from build123d import *

# Parameters (mm, degrees)
F0_R     = 1.5
F1_DEPTH = 3


with BuildPart() as f1:
    # F0 (on Top) → F1 (new body)
    with BuildSketch(Plane.XY):
        with BuildLine():
            ThreePointArc((26, 35), (22.464466, 26.464466), (31, 30))
            ThreePointArc((31, 30), (30.829629, 31.294095), (30.330127, 32.5))
            ThreePointArc((30.330127, 32.5), (28.5, 34.330127), (26, 35))
        make_face()
        with Locations((26, 30)):
            Circle(F0_R, mode=Mode.SUBTRACT)
        with BuildLine():
            ThreePointArc((30.330127, 32.5), (30.829629, 31.294095), (31, 30))
            ThreePointArc((31, 30), (22.464466, 26.464466), (26, 35))
            Line((26, 35), (-26, 35))
            ThreePointArc((-26, 35), (-22.464466, 33.535534), (-21, 30))
            ThreePointArc((-21, 30), (-27.294095, 25.170371), (-30.330127, 32.5))
            Line((-30.330127, 32.5), (-43.310889, 10.01666))
            ThreePointArc((-43.310889, 10.01666), (-37.686667, 12.34629), (-33.980762, 7.51666))
            ThreePointArc((-33.980762, 7.51666), (-37.686667, 2.687031), (-43.310889, 5.01666))
            Line((-43.310889, 5.01666), (-17.310889, -40.01666))
            ThreePointArc((-17.310889, -40.01666), (-14.274857, -32.687031), (-7.980762, -37.51666))
            ThreePointArc((-7.980762, -37.51666), (-9.445228, -41.052194), (-12.980762, -42.51666))
            Line((-12.980762, -42.51666), (12.980762, -42.51666))
            ThreePointArc((12.980762, -42.51666), (9.445228, -33.981127), (17.980762, -37.51666))
            ThreePointArc((17.980762, -37.51666), (17.810391, -38.810756), (17.310889, -40.01666))
            Line((17.310889, -40.01666), (43.310889, 5.01666))
            ThreePointArc((43.310889, 5.01666), (33.980762, 7.51666), (43.310889, 10.01666))
            Line((43.310889, 10.01666), (30.330127, 32.5))
        make_face()
        with Locations((-25.980762, -15)):
            Circle(F0_R, mode=Mode.SUBTRACT)
        with BuildLine():
            ThreePointArc((32.913325, 11.015246), (33.848011, 9.80077), (33.648709, 8.281274))
            Line((33.648709, 8.281274), (9.652561, -33.281274))
            ThreePointArc((9.652561, -33.281274), (8.43629, -34.213623), (6.91718, -34.011398))
            Line((6.91718, -34.011398), (5.99667, -33.477578))
            ThreePointArc((5.99667, -33.477578), (5.266988, -32.745787), (5, -31.747454))
            Line((5, -31.747454), (5, -30))
            ThreePointArc((5, -30), (0, -25), (-5, -30))
            Line((-5, -30), (-5, -31.747454))
            ThreePointArc((-5, -31.747454), (-5.266988, -32.745787), (-5.99667, -33.477578))
            Line((-5.99667, -33.477578), (-6.91718, -34.011398))
            ThreePointArc((-6.91718, -34.011398), (-8.43629, -34.213623), (-9.652561, -33.281274))
            Line((-9.652561, -33.281274), (-33.648709, 8.281274))
            ThreePointArc((-33.648709, 8.281274), (-33.848011, 9.80077), (-32.913325, 11.015246))
            Line((-32.913325, 11.015246), (-31.990768, 11.545521))
            ThreePointArc((-31.990768, 11.545521), (-30.992178, 11.811548), (-29.994102, 11.5436))
            Line((-29.994102, 11.5436), (-28.480762, 10.669873))
            ThreePointArc((-28.480762, 10.669873), (-21.650635, 12.5), (-23.480762, 19.330127))
            Line((-23.480762, 19.330127), (-24.994102, 20.203854))
            ThreePointArc((-24.994102, 20.203854), (-25.72519, 20.934239), (-25.994098, 21.932057))
            Line((-25.994098, 21.932057), (-25.996145, 22.996152))
            ThreePointArc((-25.996145, 22.996152), (-25.411722, 24.412853), (-23.996149, 25))
            Line((-23.996149, 25), (23.996149, 25))
            ThreePointArc((23.996149, 25), (25.411722, 24.412853), (25.996145, 22.996152))
            Line((25.996145, 22.996152), (25.994098, 21.932057))
            ThreePointArc((25.994098, 21.932057), (25.72519, 20.934239), (24.994102, 20.203854))
            Line((24.994102, 20.203854), (23.480762, 19.330127))
            ThreePointArc((23.480762, 19.330127), (21.650635, 12.5), (28.480762, 10.669873))
            Line((28.480762, 10.669873), (29.994102, 11.5436))
            ThreePointArc((29.994102, 11.5436), (30.992178, 11.811548), (31.990768, 11.545521))
            Line((31.990768, 11.545521), (32.913325, 11.015246))
        make_face(mode=Mode.SUBTRACT)
        with Locations((0, -30)):
            Circle(F0_R, mode=Mode.SUBTRACT)
        with Locations((25.980762, -15)):
            Circle(F0_R, mode=Mode.SUBTRACT)
        with Locations((-25.980762, 15)):
            Circle(F0_R, mode=Mode.SUBTRACT)
        with Locations((25.980762, 15)):
            Circle(F0_R, mode=Mode.SUBTRACT)
        with Locations((0, 30)):
            Circle(F0_R, mode=Mode.SUBTRACT)
        with BuildLine():
            ThreePointArc((43.980762, 7.51666), (43.810391, 8.810756), (43.310889, 10.01666))
            ThreePointArc((43.310889, 10.01666), (33.980762, 7.51666), (43.310889, 5.01666))
            ThreePointArc((43.310889, 5.01666), (43.810391, 6.222565), (43.980762, 7.51666))
        make_face()
        with Locations((38.980762, 7.51666)):
            Circle(F0_R, mode=Mode.SUBTRACT)
        with BuildLine():
            ThreePointArc((-21, 30), (-22.464466, 33.535534), (-26, 35))
            ThreePointArc((-26, 35), (-28.5, 34.330127), (-30.330127, 32.5))
            ThreePointArc((-30.330127, 32.5), (-27.294095, 25.170371), (-21, 30))
        make_face()
        with Locations((-26, 30)):
            Circle(F0_R, mode=Mode.SUBTRACT)
        with BuildLine():
            ThreePointArc((12.980762, -42.51666), (15.480762, -41.846788), (17.310889, -40.01666))
            ThreePointArc((17.310889, -40.01666), (17.810391, -38.810756), (17.980762, -37.51666))
            ThreePointArc((17.980762, -37.51666), (9.445228, -33.981127), (12.980762, -42.51666))
        make_face()
        with Locations((12.980762, -37.51666)):
            Circle(F0_R, mode=Mode.SUBTRACT)
        with BuildLine():
            ThreePointArc((-33.980762, 7.51666), (-37.686667, 12.34629), (-43.310889, 10.01666))
            ThreePointArc((-43.310889, 10.01666), (-43.980762, 7.51666), (-43.310889, 5.01666))
            ThreePointArc((-43.310889, 5.01666), (-37.686667, 2.687031), (-33.980762, 7.51666))
        make_face()
        with Locations((-38.980762, 7.51666)):
            Circle(F0_R, mode=Mode.SUBTRACT)
        with BuildLine():
            ThreePointArc((-17.310889, -40.01666), (-15.480762, -41.846788), (-12.980762, -42.51666))
            ThreePointArc((-12.980762, -42.51666), (-9.445228, -41.052194), (-7.980762, -37.51666))
            ThreePointArc((-7.980762, -37.51666), (-14.274857, -32.687031), (-17.310889, -40.01666))
        make_face()
        with Locations((-12.980762, -37.51666)):
            Circle(F0_R, mode=Mode.SUBTRACT)
    extrude(amount=F1_DEPTH)


solid = f1.part
Here's how the part is built. I have some questions about the finished solid (model axes, mm). A direction names the side the tool comes from. Round coordinates to 2 decimals unless told otherwise and drop trailing zeros. Write each loop counter-clockwise with the first axis right and the second up, starting at its lowest first coordinate (ties: lowest second). Pieces come first, ordered by that corner, then holes. Notation, with made-up numbers: (72, 74.5) -> (93, 74.5) arc R19 cw to (93, 88.5) -> close; hole circle Ø3 at (18, 53.25). An arc over 180 degrees is marked (long way). One line per item, written item: value.
1) Suppose I cut it at D-D on x = -19. List the corners of the cut face in (y, z) for me.
Filled sheet:
outline: (-37.09, 0) -> (-17.09, 0) -> (-17.09, 3) -> (-37.09, 3) -> close; (25, 0) -> (35, 0) -> (35, 3) -> (25, 3) -> close
2) Suppose I cut it at B-B on y = 0.5. List the corners of the cut face in (x, z) for me.
Filled sheet:
outline: (-40.7, 0) -> (-29.16, 0) -> (-29.16, 3) -> (-40.7, 3) -> close; (29.16, 0) -> (40.7, 0) -> (40.7, 3) -> (29.16, 3) -> close
3) Suppose I cut it at C-C on y = 15. List the corners of the cut face in (x, z) for me, plus the area to 3 significant figures.
Filled sheet:
outline: (-40.43, 0) -> (-27.48, 0) -> (-27.48, 3) -> (-40.43, 3) -> close; (-24.48, 0) -> (-20.98, 0) -> (-20.98, 3) -> (-24.48, 3) -> close; (20.98, 0) -> (24.48, 0) -> (24.48, 3) -> (20.98, 3) -> close; (27.48, 0) -> (40.43, 0) -> (40.43, 3) -> (27.48, 3) -> close
area: 98.7 mm2
4) For faces 1 (the face through (0, 25, 1)), 2 (the face through (36.91, 21.1, 1.48)), which set-ups out of +Z, -Z, +X, -X, +Y, -Y let a thin tool reach every point of the face, with its end or its side?
Filled sheet:
face 1: +Z, -Z
face 2: +Z, -Z, +X, +Y
5) If I drill on line 1 (X direction, y = 7, z = 2.2); line 2 (Y direction, x = -24, z = 1.45); line 3 (Y direction, x = 25, z = 1.8), over which ranges is the centre line in solid material (lowest first)? Write a range as [from, to].
Filled sheet:
line 1: x = [-43.95, -40.39], [-37.57, -32.91], [32.91, 37.57], [40.39, 43.95]
line 2: y = [-28.43, -8.43], [10.41, 19.63], [25, 35]
line 3: y = [-26.7, -16.13], [-13.87, -6.7], [10.1, 13.87], [16.13, 20.21], [24.73, 28.88], [31.12, 35]
6) I'm going to push flat-ended pins straight in: pin 1 Ø2.5 at (x, y) = (26, 30) entering from +Z; pin 2 Ø1.5 at (y, z) = (1, 0.5) entering from +X; pin 3 Ø0.5 at (y, z) = (-31, 1.5) entering from -X; pin 4 Ø1.5 at (y, z) = (-32.5, 0.5) entering from -X. Where does each tip first touch, or does it pass through?
Filled sheet:
pin 1: passes through
pin 2: stops at x = 41.42
pin 3: stops at x = -22.66
pin 4: stops at x = -22.08
7) Suppose I cut it at A-A on x = 0. List the corners of the cut face in (y, z) for me, plus the area to 4 significant figures.
Filled sheet:
outline: (-42.52, 0) -> (-31.5, 0) -> (-31.5, 3) -> (-42.52, 3) -> close; (-28.5, 0) -> (-25, 0) -> (-25, 3) -> (-28.5, 3) -> close; (25, 0) -> (28.5, 0) -> (28.5, 3) -> (25, 3) -> close; (31.5, 0) -> (35, 0) -> (35, 3) -> (31.5, 3) -> close
area: 64.55 mm2
8) We'd pull the mould along Y, two halves only. Please class faces 3 (the face through (8.458, -34.208, 1.479)), 4 (the face through (-36.73, 21.416, 1.479)), 5 (the face through (15.449, -41.865, 1.479)), 6 (the face through (-23, 14, 0)): released by +Y, released by -Y, zero draft, split by the parting line, or undercut.
Filled sheet:
face 3: undercut
face 4: released by +Y
face 5: released by -Y
face 6: zero draft
